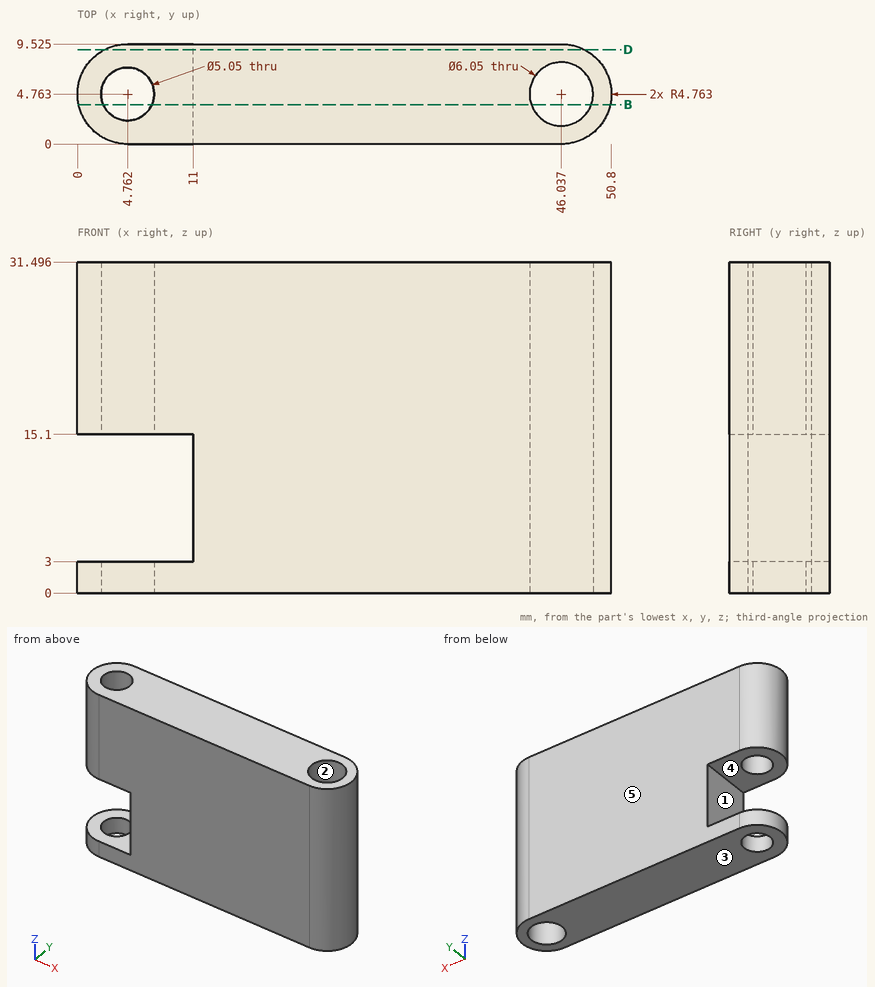
Geometry: see drawing. Coordinates: mm, zero at the bounding-box minimum. A direction names the side the tool comes from. Give positions to 0.01 mm unless a question says otherwise; leave off trailing zeros. Loops run counter-clockwise (first coordinate to the right, second up) from the corner with the lowest first, then second, coordinate; pieces in that order, holes last. Notation, with made-up numbers: (-16, 4) -> (40, 4) arc R19 cw to (40, 35) -> close; hole circle Ø9 at (63, -18). An arc over 180 degrees is marked (long way). Put each result on its own line as item: value.
1. Cut plane D-D (y = 9). Return the cut outline in (x, z) (1 decimal).
Taken from the geometry:
outline: (2.6, 0) -> (48.2, 0) -> (48.2, 31.5) -> (2.6, 31.5) -> (2.6, 15.1) -> (11, 15.1) -> (11, 3) -> (2.6, 3) -> close
2. Pull-direction query (Z, two-part tool) for the marked faces 1, 2 and 3; classes: released by +Z, released by -Z, zero draft, split by the parting line, or undercut.
Taken from the geometry:
face 1: undercut
face 2: zero draft
face 3: released by -Z
3. Cut plane B-B (y = 3.75). Count the separate pieces of the cut face and the enclosed holes in it, plus the area to 3 significant figures.
Taken from the geometry:
separate pieces: 4
enclosed holes: 0
area: 1,190 mm2
4. Pin query (flat end, axial travel): P1, Ø4.5, axis at x = 4.76, y = 4.76, coming from the -Z side; P2, Ø2, axis at y = 2, z = 10.5, coming from the +X side. Return the tip coordinate at first contact, or that it passes through.
Taken from the geometry:
P1: passes through
P2: stops at x = 50.46
5. Ray query, line 1 along X through (y, z) = (5.5, 29) (1 decimal); line 2 along X through (y, z) = (3, 23) (1 decimal); line 3 along Z through (x, y) = (2, 1.5) (1 decimal). Return the intervals inside material, ascending. Write a range as [from, to].
Taken from the geometry:
line 1: x = [0.1, 2.3], [7.2, 43.1], [49, 50.7]
line 2: x = [0.3, 3], [6.6, 43.6], [48.5, 50.5]
line 3: z = [0, 3], [15.1, 31.5]
6. Set-up query: the marked faces 4 and 5. Return all of +Z, -Z, +X, -X, +Y, -Y with unobstructed straight access to the full face (end or side cutting, diameter ignored); none if empty.
Taken from the geometry:
face 4: -X, +Y, -Y
face 5: +Z, -Z, +X, -X, +Y
